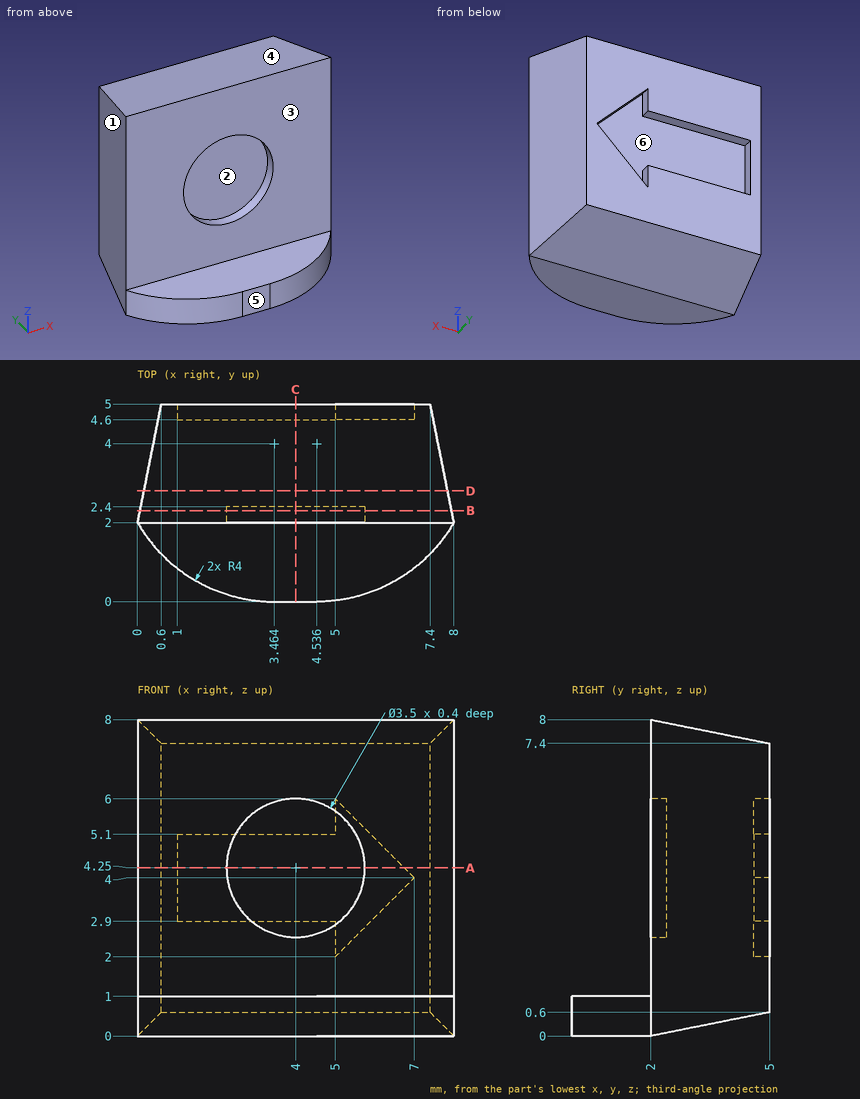
The drawing under review shows one solid part. Ordinate dimensions are in mm from its lowest x, y, z. A direction names the side the tool comes from. Coordinates: 2 decimals unless noted, no trailing zeros. Order: outer loops, then holes, each group sorted by start corner. A loop starts at its lowest first (then second) coordinate and runs counter-clockwise, first axis right, second up. Notation, with made-up numbers: (69.5, 58.25) -> (116.5, 58.25) arc R17 cw to (116.5, 89.25) -> close; hole circle Ø5 at (-3.75, 24.5). An arc over 180 degrees is marked (long way). Return JSON: item names as keys, results as strings.
1. We need section D-D on y = 2.8. Write out the cut boundary in (x, z), and give its area (3 significant figures).
Answer block:
{"outline": "(0.16, 0.16) -> (7.84, 0.16) -> (7.84, 7.84) -> (0.16, 7.84) -> close", "area": "59.0 mm²"}
2. We need section A-A on z = 4.25. Write out the cut boundary in (x, y), and give its area (3 significant figures).
Answer block:
{"outline": "(0, 2) -> (2.25, 2) -> (2.25, 2.4) -> (5.75, 2.4) -> (5.75, 2) -> (8, 2) -> (7.4, 5) -> (6.75, 5) -> (6.75, 4.6) -> (1, 4.6) -> (1, 5) -> (0.6, 5) -> close", "area": "18.5 mm²"}
3. The part is to be moulded in two halves that separate along Z. For the marked faces 4, 5 and 6, say which applies: +Z half, -Z half, draft (parallel to the pull), parting line (faces both ways), or undercut.
Answer block:
{"face 4": "+Z half", "face 5": "draft", "face 6": "undercut"}
4. For pin 1 Ø3 at (x, z) = (4, 4.25) entering from -Y; pin 2 Ø1.5 at (x, y) = (2, 0.5) entering from +Z; pin 3 Ø4 at (x, z) = (3.5, 5) entering from -Y, all flat-tipped, find the tip position at first contact; note any pin that passes through.
Answer block:
{"pin 1": "y = 2.4", "pin 2": "z = 1", "pin 3": "y = 2"}
5. For line 1 (Z direction, x = 3.5, y = 1.75); line 2 (Y direction, x = 6, z = 6.5); line 3 (X direction, y = 2.2, z = 4.25), list the stretches that pass through material, from the lowest coordinate up. Write a range as from..to.
Answer block:
{"line 1": "0..1", "line 2": "2..5", "line 3": "0.04..2.25, 5.75..7.96"}
6. We need section B-B on y = 2.3. Write out the cut boundary in (x, z).
Answer block:
{"outline": "(0.06, 0.06) -> (7.94, 0.06) -> (7.94, 7.94) -> (0.06, 7.94) -> close; hole circle Ø3.5 at (4, 4.25)"}
7. Machinability: for the marked faces 1, 2 and 3, which of the approach directions +Z, -Z, +X, -X, +Y, -Y give a long, thin tool a straight path to every point of the face, cutting with its end or side? Answer none if there is none.
Answer block:
{"face 1": "+Z, -Z, -X, +Y", "face 2": "-Y", "face 3": "+Z, +X, -X, -Y"}
8. We need section C-C on x = 4. Write out the cut boundary in (y, z).
Answer block:
{"outline": "(0, 0) -> (2, 0) -> (5, 0.6) -> (5, 2.9) -> (4.6, 2.9) -> (4.6, 5.1) -> (5, 5.1) -> (5, 7.4) -> (2, 8) -> (2, 6) -> (2.4, 6) -> (2.4, 2.5) -> (2, 2.5) -> (2, 1) -> (0, 1) -> close"}
